Work out the finished part from the listing and answer in its coordinate system (mm). A direction names the side the tool comes from. Give positions to 0.01 mm unless a question says otherwise; leave off trailing zeros. Loops run counter-clockwise (first coordinate to the right, second up) from the corner with the lowest first, then second, coordinate; pieces in that order, holes last. Notation, with made-up numbers: (74.25, 34.5) - (89.25, 34.5) arc R28 ccw to (89.25, 69.5) - close; hole circle Ø3 at (56.25, 44). An arc over 180 degrees is marked (long way). Use CSV: the item, a comma, the result in double quotes.
from build123d import *

# Parameters (mm, degrees)
SKETCH1_W           = 4
SKETCH1_H           = 4
SKETCH1_W_2         = 92.25
SKETCH1_H_2         = 64.75
BOSS_EXTRUDE1_DEPTH = 4
SKETCH1_3_W         = 4
SKETCH1_3_H         = 4
BOSS_EXTRUDE2_DEPTH = 21
CUT_EXTRUDE1_DEPTH  = 21
SKETCH2_4_R         = 2
CUT_EXTRUDE3_DEPTH  = 21
SKETCH5_W           = 4
SKETCH5_H           = 4
BOSS_EXTRUDE3_DEPTH = 9.5
SKETCH7_W           = 4
SKETCH7_H           = 4
BOSS_EXTRUDE4_DEPTH = 20
CUT_EXTRUDE4_DEPTH  = 10
SKETCH10_W          = 5.918371549
SKETCH10_H          = 22.91291731
CUT_EXTRUDE5_DEPTH  = 10


with BuildPart() as part:
    # Sketch1 → Boss-Extrude1 (new body)
    with BuildSketch(Plane(origin=(0, 0, 0), x_dir=(1, 0, 0), z_dir=(0, 1, 0))):
        Polygon((54.335861322, 29.953412784), (-41.914138678, 29.953412784), (-41.914138678, 25.953412784), (50.335861322, 25.953412784), (50.335861322, -38.796587216), (54.335861322, -38.796587216), align=None)
        with Locations((-43.914138678, 27.953412784)):
            Rectangle(SKETCH1_W, SKETCH1_H)
        Polygon((-41.914138678, -38.796587216), (-41.914138678, 25.953412784), (-45.914138678, 25.953412784), (-45.914138678, -42.796587216), (50.335861322, -42.796587216), (50.335861322, -38.796587216), align=None)
        with Locations((52.335861322, -40.796587216)):
            Rectangle(SKETCH1_W, SKETCH1_H)
        with Locations((4.210861322, -6.421587216)):
            Rectangle(SKETCH1_W_2, SKETCH1_H_2)
    extrude(amount=BOSS_EXTRUDE1_DEPTH)

    # Sketch1_3 → Boss-Extrude2 (add)
    with BuildSketch(Plane(origin=(0, 0, 0), x_dir=(1, 0, 0), z_dir=(0, 1, 0))):
        Polygon((54.335861322, 29.953412784), (-41.914138678, 29.953412784), (-41.914138678, 25.953412784), (50.335861322, 25.953412784), (50.335861322, -38.796587216), (54.335861322, -38.796587216), align=None)
        with Locations((-43.914138678, 27.953412784)):
            Rectangle(SKETCH1_3_W, SKETCH1_3_H)
        Polygon((-41.914138678, -38.796587216), (-41.914138678, 25.953412784), (-45.914138678, 25.953412784), (-45.914138678, -42.796587216), (50.335861322, -42.796587216), (50.335861322, -38.796587216), align=None)
        with Locations((52.335861322, -40.796587216)):
            Rectangle(SKETCH1_3_W, SKETCH1_3_H)
    extrude(amount=BOSS_EXTRUDE2_DEPTH)

    # Sketch2 → Cut-Extrude1 (cut)
    with BuildSketch(Plane.XZ):
        Polygon((4.210861322, 17.921587216), (4.210861322, 6.421587216), (5.878483504, 5.211417502), (7.210861322, 17.921587216), align=None)
        Polygon((1.210861322, 17.921587216), (1.210861322, 8.598644572), (4.210861322, 6.421587216), (4.210861322, 17.921587216), align=None)
        Polygon((4.210861322, 6.421587216), (1.210861322, 8.598644572), (1.210861322, -4.953073118), (4.812963363, -4.953073118), (5.878483504, 5.211417502), align=None)
    extrude(amount=-CUT_EXTRUDE1_DEPTH, mode=Mode.SUBTRACT)

    # Sketch2_4 → Cut-Extrude3 (cut)
    with BuildSketch(Plane.XZ):
        with Locations((-31.414677441, 6.546582571)):
            Circle(SKETCH2_4_R)
    extrude(amount=-CUT_EXTRUDE3_DEPTH, mode=Mode.SUBTRACT)

    # Sketch5 → Boss-Extrude3 (add)
    with BuildSketch(Plane(origin=(0, 0, 0), x_dir=(-1, 0, 0), z_dir=(0, -1, 0))):
        with Locations((-10.710861322, -23.921587216)):
            Rectangle(SKETCH5_W, SKETCH5_H)
        with Locations((2.289138678, -24.046587216)):
            Rectangle(SKETCH5_W, SKETCH5_H)
    extrude(amount=BOSS_EXTRUDE3_DEPTH)

    # Sketch7 → Boss-Extrude4 (add)
    with BuildSketch(Plane(origin=(0, 0, 22.046587216), x_dir=(-1, 0, 0), z_dir=(0, 0, -1))):
        with Locations((2.289138678, -7.5)):
            Rectangle(SKETCH7_W, SKETCH7_H)
        with Locations((-10.710861322, -7.5)):
            Rectangle(SKETCH7_W, SKETCH7_H)
    extrude(amount=BOSS_EXTRUDE4_DEPTH)

    # Sketch8 → Cut-Extrude4 (cut)
    with BuildSketch(Plane(origin=(0, 0, -29.953412784), x_dir=(-1, 0, 0), z_dir=(0, 0, -1))):
        Polygon((-4.443587371, 21), (-4.443587371, 10.548750594), (1.289138678, 9.347880299), (1.289138678, 21), (-4.210861322, 21), align=None)
        Polygon((-9.943587371, 21), (-9.943587371, 11.700870295), (-4.443587371, 10.548750594), (-4.443587371, 21), align=None)
        Polygon((-4.443587371, 10.548750594), (-9.943587371, 11.700870295), (-9.943587371, 4), (1.289138678, 4), (1.289138678, 9.347880299), align=None)
    extrude(amount=-CUT_EXTRUDE4_DEPTH, mode=Mode.SUBTRACT)

    # Sketch10 → Cut-Extrude5 (cut)
    with BuildSketch(Plane.XZ):
        with Locations((4.170047097, 6.465128561)):
            Rectangle(SKETCH10_W, SKETCH10_H)
    extrude(amount=-CUT_EXTRUDE5_DEPTH, mode=Mode.SUBTRACT)


solid = part.part
Item 1: Given P1, Ø1.2, axis at x = 9.5, y = -2, coming from the -Z side; P2, Ø1, axis at x = -35.5, z = 27.5, coming from the +Y side; P3, Ø1.2, axis at x = -1.5, y = -3, coming from the -Z side, each flat-ended and moving along its own axis, determine where each tip first touches the part or whether it passes through.
Determined:
P1,"stops at z = 21.92"
P2,"stops at y = 4"
P3,"stops at z = 22.05"
Item 2: A cutting plane is placed at A-A on z = -19. Determine the outline of the cut face in (x, y).
Determined:
outline,"(-45.91, 0) - (54.34, 0) - (54.34, 21) - (50.34, 21) - (50.34, 4) - (-41.91, 4) - (-41.91, 21) - (-45.91, 21) - close"
Item 3: A cutting plane is placed at D-D on y = 8. Determine the outline of the cut face in (x, z).
Determined:
outline,"(-45.91, -29.95) - (-1.29, -29.95) - (-1.29, -25.95) - (-41.91, -25.95) - (-41.91, 38.8) - (50.34, 38.8) - (50.34, -25.95) - (9.94, -25.95) - (9.94, -29.95) - (54.34, -29.95) - (54.34, 42.8) - (-45.91, 42.8) - close"
Item 4: For faces 1 (the flat face through (11, -7, 2.047)), 2 (the flat face through (30, 12, -25.953)), 3 (the flat face through (-0.289, -7, 17)), 4 (the flat face through (-4.289, -7, 17)), determine the directions among +Z, -Z, +X, -X, +Y, -Y from which every point of the face is accessible in a straight line to the end or side of a thin tool.
Determined:
face 1,"-Z, +X, -X, -Y"
face 2,"+Y"
face 3,"+Z, -Z, -Y"
face 4,"+Z, -Z, -X, -Y"
Item 5: A cutting plane is placed at B-B on y = -1.5. Determine the outline of the cut face in (x, z).
Determined:
outline,"(-4.29, 22.05) - (-0.29, 22.05) - (-0.29, 26.05) - (-4.29, 26.05) - close; (8.71, 21.92) - (12.71, 21.92) - (12.71, 25.92) - (8.71, 25.92) - close"
Item 6: The mould has two halves that part along Z. Classify faces 5 (the flat face through (4, 2, -4.991)), 6 (the flat face through (5, 12, 38.797)), 7 (the flat face through (-2, -7, 2.047)), 8 (the flat face through (54.336, 10, 7)): pulls with the +Z half, pulls with the -Z half, needs draft (parallel to the pull), parting line crosses it, or undercut.
Determined:
face 5,"undercut"
face 6,"undercut"
face 7,"pulls with the -Z half"
face 8,"needs draft"
Item 7: Find the intervals of material crossed by line 1 (X direction, y = 18, z = -7); line 2 (Z direction, x = 16.5, y = 8.5); line 3 (X direction, y = -6, z = 14), in increasing order.
Determined:
line 1,"x = -45.91 to -41.91, 50.34 to 54.34"
line 2,"z = -29.95 to -25.95, 38.8 to 42.8"
line 3,"x = -4.29 to -0.29, 8.71 to 12.71"
Item 8: A cutting plane is placed at C-C on x = 47.5. Determine the outline of the cut face in (y, z), and give its area (3 significant figures).
Determined:
outline,"(0, -29.95) - (21, -29.95) - (21, -25.95) - (4, -25.95) - (4, 38.8) - (21, 38.8) - (21, 42.8) - (0, 42.8) - close"
area,"427 mm²"
